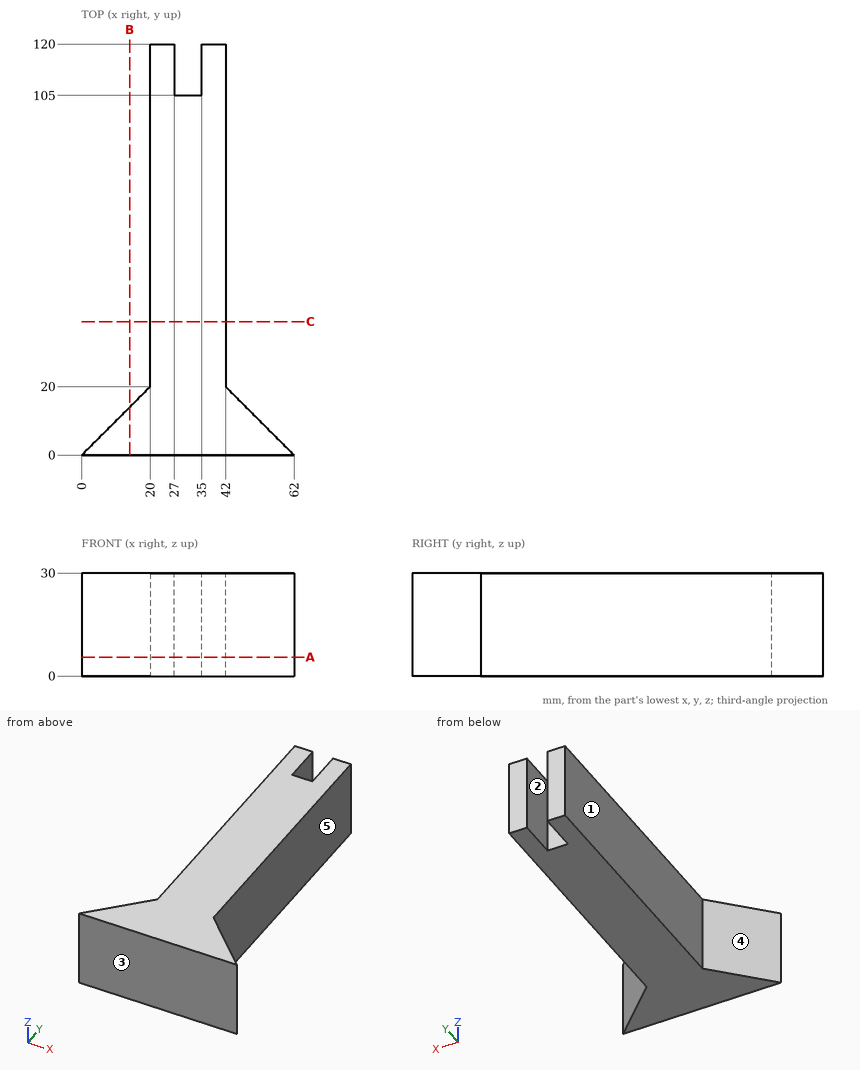
Geometry: see drawing. Coordinates: mm, zero at the bounding-box minimum. A direction names the side the tool comes from. Coordinates: 2 decimals unless noted, no trailing zeros. Loops run counter-clockwise (first coordinate to the right, second up) from the corner with the lowest first, then second, coordinate; pieces in that order, holes last.
(1) Set-up query: the marked faces 4 and 5. Return all of +Z, -Z, +X, -X, +Y, -Y with unobstructed straight access to the full face (end or side cutting, diameter ignored); none if empty.
(2) First-contact query: pin 1 Ø12 at (y, z) = (91, 24) entering from +X; pin 2 Ø6.5 at (x, z) = (29.5, 16) entering from +Y; pin 3 Ø2 at (y, z) = (107.5, 19) entering from -X. Flat tips, straight axial feed; report the tip coordinate or a pass-through.
(3) Section C-C on y = 39. Return the cut outline in (x, z).
(4) Section B-B on x = 14. Return the cut outline in (y, z).
(5) Material intervals for probe 1 along X at (y, z) = (113.5, 7); probe 2 along X at (y, z) = (48, 2.5); probe 3 along Y at (x, z) = (30.5, 18.25), sorted ascending.
(6) Section A-A on z = 5.5. Return the cut outline in (x, y), then the cut area to 3 significant figures.
(7) Pull-direction query (X, two-part tool) for the marked faces 1, 2 and 3; classes: released by +X, released by -X, zero draft, split by the parting line, or undercut.
Data:
1. face 4: +Z, -Z, -X, +Y
1. face 5: +Z, -Z, +X, +Y
2. pin 1: stops at x = 42
2. pin 2: stops at y = 120
2. pin 3: stops at x = 20
3. outline: (20, 0) - (42, 0) - (42, 30) - (20, 30) - close
4. outline: (0, 0) - (14, 0) - (14, 30) - (0, 30) - close
5. probe 1: x = 20 to 27, 35 to 42
5. probe 2: x = 20 to 42
5. probe 3: y = 0 to 105
6. outline: (0, 0) - (62, 0) - (42, 20) - (42, 120) - (35, 120) - (35, 105) - (27, 105) - (27, 120) - (20, 120) - (20, 20) - close
6. area: 2,920 mm2
7. face 1: released by -X
7. face 2: undercut
7. face 3: zero draft
